The model under review builds one solid part; all positions refer to its coordinate system, in mm. A direction names the side the tool comes from. Give positions to 0.01 mm unless a question says otherwise; leave off trailing zeros. Loops run counter-clockwise (first coordinate to the right, second up) from the corner with the lowest first, then second, coordinate; pieces in that order, holes last. Notation, with made-up numbers: (33.25, -13.75) - (88.25, -13.75) arc R19 cw to (88.25, 21.25) - close; hole circle Ø7 at (6.5, 76.5). An arc over 180 degrees is marked (long way). Answer as a JSON object with one key per item and string values.
from build123d import *

# Parameters (mm, degrees)
F0_W     = 24
F0_H     = 24
F1_DEPTH = 26
F2_R     = 1.85
F3_DEPTH = 7.5
F5_START = -3.81
F4_R     = 1.85
F5_DEPTH = 3.19
F6_DEPTH = 2


with BuildPart() as f1:
    # F0 (on Top) → F1 (new body)
    with BuildSketch(Plane.XY):
        Rectangle(F0_W, F0_H)
        with BuildLine():
            Line((-10.2, -8.7), (-10.2, -8.6))
            Line((-10.2, -8.6), (-10.2, -2.5))
            Line((-10.2, -2.5), (-6.2, -2.5))
            ThreePointArc((-6.2, -2.5), (-5.4928932188, -2.2071067812), (-5.2, -1.5))
            Line((-5.2, -1.5), (-5.2, 1.5))
            ThreePointArc((-5.2, 1.5), (-5.4928932188, 2.2071067812), (-6.2, 2.5))
            Line((-6.2, 2.5), (-10.2, 2.5))
            Line((-10.2, 2.5), (-10.2, 8.7))
            ThreePointArc((-10.2, 8.7), (-9.7606601718, 9.7606601718), (-8.7, 10.2))
            Line((-8.7, 10.2), (-8.6, 10.2))
            Line((-8.6, 10.2), (-2.5, 10.2))
            Line((-2.5, 10.2), (-2.5, 6.2))
            ThreePointArc((-2.5, 6.2), (-2.2071067812, 5.4928932188), (-1.5, 5.2))
            Line((-1.5, 5.2), (1.5, 5.2))
            ThreePointArc((1.5, 5.2), (2.2071067812, 5.4928932188), (2.5, 6.2))
            Line((2.5, 6.2), (2.5, 10.2))
            Line((2.5, 10.2), (8.7, 10.2))
            ThreePointArc((8.7, 10.2), (9.7606601718, 9.7606601718), (10.2, 8.7))
            Line((10.2, 8.7), (10.2, 8.6))
            Line((10.2, 8.6), (10.2, 2.5))
            Line((10.2, 2.5), (6.2, 2.5))
            ThreePointArc((6.2, 2.5), (5.4928932188, 2.2071067812), (5.2, 1.5))
            Line((5.2, 1.5), (5.2, -1.5))
            ThreePointArc((5.2, -1.5), (5.4928932188, -2.2071067812), (6.2, -2.5))
            Line((6.2, -2.5), (10.2, -2.5))
            Line((10.2, -2.5), (10.2, -8.7))
            ThreePointArc((10.2, -8.7), (9.7606601718, -9.7606601718), (8.7, -10.2))
            Line((8.7, -10.2), (8.6, -10.2))
            Line((8.6, -10.2), (2.5, -10.2))
            Line((2.5, -10.2), (2.5, -6.2))
            ThreePointArc((2.5, -6.2), (2.2071067812, -5.4928932188), (1.5, -5.2))
            Line((1.5, -5.2), (-1.5, -5.2))
            ThreePointArc((-1.5, -5.2), (-2.2071067812, -5.4928932188), (-2.5, -6.2))
            Line((-2.5, -6.2), (-2.5, -10.2))
            Line((-2.5, -10.2), (-8.7, -10.2))
            ThreePointArc((-8.7, -10.2), (-9.7606601718, -9.7606601718), (-10.2, -8.7))
        make_face(mode=Mode.SUBTRACT)
    extrude(amount=F1_DEPTH)

    # F2 (on face) → F3 (cut)
    with BuildSketch(Plane.XZ.offset(12)):
        with Locations((0, 53)):
            Circle(F2_R)
        with Locations((8, 45)):
            Circle(F2_R)
        with Locations((-8, 45)):
            Circle(F2_R)
        with Locations((0, 37)):
            Circle(F2_R)
        with Locations((-8, 29)):
            Circle(F2_R)
        with Locations((0, 21)):
            Circle(F2_R)
        with Locations((8, 29)):
            Circle(F2_R)
        with Locations((8, 13)):
            Circle(F2_R)
        with Locations((-8, 13)):
            Circle(F2_R)
        with Locations((0, 5)):
            Circle(F2_R)
    extrude(amount=-F3_DEPTH, mode=Mode.SUBTRACT)

    # F4 (on face) → F5 (cut)
    with BuildSketch(Plane.XZ.offset(12).offset(F5_START)):
        Polygon((1.3331978443, 18.6901357984), (2.0000989222, 19.8448934496), (2.667, 19.8448934496), (2.667, 22.1545832015), (2.0004010778, 22.1545832015), (1.3338021557, 23.3095153022), (-1.3331978443, 23.3098642016), (-2.0004011691, 22.1545832015), (-2.667, 22.1545832015), (-2.667, 19.8448934496), (-2.0000989222, 19.8448934496), (-1.3338021557, 18.6904846978), align=None)
        with Locations((0, 21)):
            Circle(F4_R, mode=Mode.SUBTRACT)
        Polygon((2.667, 6.1551065504), (2.0000989222, 6.1551065504), (1.3331978443, 7.3098642016), (-1.3338021557, 7.3095153022), (-2.0000989906, 6.15510659), (-2.667, 6.1551065504), (-2.667, 3.8454167985), (-2.0004011691, 3.8454167985), (-1.3331978443, 2.6901357984), (1.3338021557, 2.6904846978), (2.0004010778, 3.8454167985), (2.667, 3.8454167985), align=None)
        with Locations((0, 5)):
            Circle(F4_R, mode=Mode.SUBTRACT)
    extrude(amount=-F5_DEPTH, mode=Mode.SUBTRACT)

    # F6 (add): a face of the model
    f6_faces = [f1.faces().sort_by_distance(p)[0] for p in [
        (0, -12, 13),
    ]]
    extrude(f6_faces, amount=F6_DEPTH)


solid = f1.part
Q1. For faces 4 (the face through (-1.662, -6.716, 6.74)), 5 (the face through (-2.215, 5.501, 12.818)), list the 3-axis set-ups (+Z, -Z, +X, -X, +Y, -Y) from which the entire face can be reached by the end or side of a thin tool; tool diameter is ignored.
Results:
{"face 4": "none", "face 5": "+Z, -Z"}
Q2. To check wall thickness, follow probe 1 along Z at (x, y) = (0, -12.6); probe 2 along Y at (x, z) = (7.5, 21.5); probe 3 along X at (y, z) = (7.5, 9.25). State the ranges of each line that lie inside material, in increasing order. Write a range as [from, to].
Results:
{"probe 1": "z = [0, 3.15], [6.85, 19.15], [22.85, 26]", "probe 2": "y = [-14, -10.2], [-2.5, 2.5], [10.2, 12]", "probe 3": "x = [-12, -10.2], [-2.5, 2.5], [10.2, 12]"}
Q3. Clearance check with a flat-ended pin moving along its axis: pin 1 Ø0.5 at (x, y) = (2, -7) entering from -Z. State where the tip first meets the part, or that it passes through.
Results:
{"pin 1": "stops at z = 0"}
Q4. Consider section D-D, the plane x = -4.5. State the section outline as (y, z) points.
Results:
{"outline": "(-14, 0) - (-10.2, 0) - (-10.2, 26) - (-14, 26) - close; (10.2, 0) - (12, 0) - (12, 26) - (10.2, 26) - close"}
Q5. Consider section C-C, the plane y = -3. State the section outline as (x, z) points, plus the area to 3 significant figures.
Results:
{"outline": "(-12, 0) - (-10.2, 0) - (-10.2, 26) - (-12, 26) - close; (10.2, 0) - (12, 0) - (12, 26) - (10.2, 26) - close", "area": "93.6 mm^2"}
Q6. Consider section B-B, the plane x = -8. State the section outline as (y, z) points.
Results:
{"outline": "(-14, 0) - (-10.2, 0) - (-10.2, 11.15) - (-14, 11.15) - close; (-14, 14.85) - (-10.2, 14.85) - (-10.2, 26) - (-14, 26) - close; (-2.5, 0) - (2.5, 0) - (2.5, 26) - (-2.5, 26) - close; (10.2, 0) - (12, 0) - (12, 26) - (10.2, 26) - close"}
Q7. The part is to be moulded in two halves that separate along X. For faces 1 (the face through (12, -1, 13)), 2 (the face through (-2.199, -5.485, 12.904)), 3 (the face through (-6, -1, 0)), say which applies: +X half, -X half, draft (parallel to the pull), parting line (faces both ways), or undercut.
Results:
{"face 1": "+X half", "face 2": "undercut", "face 3": "draft"}
Q8. Consider section A-A, the plane y = 7. State the section outline as (x, z) points, plus the area to 3 significant figures.
Results:
{"outline": "(-12, 0) - (-10.2, 0) - (-10.2, 26) - (-12, 26) - close; (-2.5, 0) - (2.5, 0) - (2.5, 26) - (-2.5, 26) - close; (10.2, 0) - (12, 0) - (12, 26) - (10.2, 26) - close", "area": "224 mm^2"}
